from build123d import *

# Parameters (mm, degrees)
SKETCH1_R           = 4
SKETCH1_R_2         = 18
BOSS_EXTRUDE1_DEPTH = 6.35
CUT_EXTRUDE1_DEPTH  = 5.08
FILLET1_R           = 2.54


with BuildPart() as part:
    # Sketch1 → Boss-Extrude1 (new body)
    with BuildSketch(Plane.XY):
        with BuildLine():
            Line((-34.561724138, 11.41740884), (-11.123448276, 22.834817679))
            ThreePointArc((-11.123448276, 22.834817679), (0, 25.4), (11.123448276, 22.834817679))
            Line((11.123448276, 22.834817679), (34.561724138, 11.41740884))
            ThreePointArc((34.561724138, 11.41740884), (41.7, 0), (34.561724138, -11.41740884))
            Line((34.561724138, -11.41740884), (11.123448276, -22.834817679))
            ThreePointArc((11.123448276, -22.834817679), (0, -25.4), (-11.123448276, -22.834817679))
            Line((-11.123448276, -22.834817679), (-34.561724138, -11.41740884))
            ThreePointArc((-34.561724138, -11.41740884), (-41.7, 0), (-34.561724138, 11.41740884))
        make_face()
        with Locations((-29, 0)):
            Circle(SKETCH1_R, mode=Mode.SUBTRACT)
        with Locations((29, 0)):
            Circle(SKETCH1_R, mode=Mode.SUBTRACT)
        Circle(SKETCH1_R_2, mode=Mode.SUBTRACT)
    extrude(amount=BOSS_EXTRUDE1_DEPTH)

    # Sketch2 → Cut-Extrude1 (cut)
    with BuildSketch(Plane(origin=(0, 0, 0), x_dir=(-1, 0, 0), z_dir=(0, 0, -1))):
        with BuildLine():
            Line((34.005551724, 10.275667956), (10.567275862, 21.693076795))
            ThreePointArc((10.567275862, 21.693076795), (0, 24.13), (-10.567275862, 21.693076795))
            Line((-10.567275862, 21.693076795), (-34.005551724, 10.275667956))
            ThreePointArc((-34.005551724, 10.275667956), (-40.43, 0), (-34.005551724, -10.275667956))
            Line((-34.005551724, -10.275667956), (-10.567275862, -21.693076795))
            ThreePointArc((-10.567275862, -21.693076795), (0, -24.13), (10.567275862, -21.693076795))
            Line((10.567275862, -21.693076795), (34.005551724, -10.275667956))
            ThreePointArc((34.005551724, -10.275667956), (40.43, 0), (34.005551724, 10.275667956))
        make_face()
    extrude(amount=-CUT_EXTRUDE1_DEPTH, mode=Mode.SUBTRACT)

    # Fillet1
    fillet1_edges = [part.edges().sort_by_distance(p)[0] for p in [
        (-41.7, 0, 6.35),
        (-22.842586207, -17.12611326, 6.35),
        (0, -25.4, 6.35),
        (22.842586207, -17.12611326, 6.35),
        (41.7, 0, 6.35),
        (22.842586207, 17.12611326, 6.35),
        (0, 25.4, 6.35),
        (0, 24.13, 5.08),
        (-22.286413793, 15.984372376, 5.08),
        (-40.43, 0, 5.08),
        (-22.286413793, -15.984372376, 5.08),
        (0, -24.13, 5.08),
        (22.286413793, -15.984372376, 5.08),
        (40.43, 0, 5.08),
        (22.286413793, 15.984372376, 5.08),
        (-22.842586207, 17.12611326, 6.35),
    ]]
    fillet(fillet1_edges, radius=FILLET1_R)


solid = part.part
The listing builds one solid part. Answer for the finished solid, in the listing's coordinates (mm). A direction names the side the tool comes from. Round coordinates to 2 decimals unless told otherwise and drop trailing zeros. Order: outer loops, then holes, each group sorted by start corner. A loop starts at its lowest first (then second) coordinate and runs counter-clockwise, first axis right, second up. Notation, with made-up numbers: (-6, 39.5) - (19, 39.5) arc R25 cw to (19, 59.5) - close; hole circle Ø2 at (0, 1.5). An arc over 180 degrees is marked (long way). Write item = value, one per line. Start each with the question number.
1) Section A-A, the plane y = 0 is taken. Write down the section's boundary in (x, z), plus the area to 3 significant figures.
2) Section C-C, the plane x = 0 is taken. Write down the section's boundary in (y, z).
3) For a pull along X with two mould halves and no side action, classify faces 1 (the cylindrical face through (-2.343, 17.847, 5.706)), 2 (the cylindrical face through (-22.689, -16.395, 5.586)), 3 (the flat face through (13, 21, 0)) as released by +X, released by -X, zero draft, split by the parting line, or undercut.
4) Straight lines are drawn through the part: L1, parallel to X at y = 0, z = 6; L2, parallel to X at y = 0, z = 5.85; L3, parallel to Z at x = 5, y = -19.5. For each, find the intervals that lie inside material, in ascending order.
5) Given pin 1 (3 mm diameter, centred on x = -5.5, y = 20, fed in from -Z); pin 2 (1.5 mm diameter, centred on y = 3.5, z = 2, fed in from -X); pin 3 (9 mm diameter, centred on x = 29, y = 0, fed in from -Z), each flat-ended and moving along its own axis, determine where each tip first touches the part or whether it passes through.
6) For faces 4 (the cylindrical face through (-41.7, -0.2, 1.9)), 5 (the cylindrical face through (40.43, 0.18, 1.25)), determine the directions among +Z, -Z, +X, -X, +Y, -Y from which every point of the face is accessible in a straight line to the end or side of a thin tool.
7) Section B-B, the plane z = 1.5 is taken. Write down the section's boundary in (x, y).
Results list:
q1.outline = (-41.7, 0) - (-40.43, 0) - (-40.43, 2.54) arc R2.54 cw to (-37.89, 5.08) - (-33, 5.08) - (-33, 6.35) - (-39.16, 6.35) arc R2.54 ccw to (-41.7, 3.81) - close; (-25, 5.08) - (-18, 5.08) - (-18, 6.35) - (-25, 6.35) - close; (18, 5.08) - (25, 5.08) - (25, 6.35) - (18, 6.35) - close; (33, 5.08) - (37.89, 5.08) arc R2.54 cw to (40.43, 2.54) - (40.43, 0) - (41.7, 0) - (41.7, 3.81) arc R2.54 ccw to (39.16, 6.35) - (33, 6.35) - close
q1.area = 52.8 mm^2
q2.outline = (-25.4, 0) - (-24.13, 0) - (-24.13, 2.54) arc R2.54 cw to (-21.59, 5.08) - (-18, 5.08) - (-18, 6.35) - (-22.86, 6.35) arc R2.54 ccw to (-25.4, 3.81) - close; (18, 5.08) - (21.59, 5.08) arc R2.54 cw to (24.13, 2.54) - (24.13, 0) - (25.4, 0) - (25.4, 3.81) arc R2.54 ccw to (22.86, 6.35) - (18, 6.35) - close
q3.face_1 = undercut
q3.face_2 = released by -X
q3.face_3 = zero draft
q4.L1 = -40.45 to -33, -25 to -18, 18 to 25, 33 to 40.45
q4.L2 = -40.67 to -33, -25 to -18, 18 to 25, 33 to 40.67
q4.L3 = 5.08 to 6.35
q5.pin_1 = 4.99
q5.pin_2 = -41.4
q5.pin_3 = 5.08
q6.face_4 = +Z, -Z, -X
q6.face_5 = -Z
q7.outline = (-34.56, -11.42) - (-11.12, -22.83) arc R25.4 ccw to (11.12, -22.83) - (34.56, -11.42) arc R12.7 ccw to (34.56, 11.42) - (11.12, 22.83) arc R25.4 ccw to (-11.12, 22.83) - (-34.56, 11.42) arc R12.7 ccw to start; hole (-34.01, -10.28) - (-10.57, -21.69) arc R24.13 ccw to (10.57, -21.69) - (34.01, -10.28) arc R11.43 ccw to (34.01, 10.28) - (10.57, 21.69) arc R24.13 ccw to (-10.57, 21.69) - (-34.01, 10.28) arc R11.43 ccw to start
